Here's the drawing with two shaded views (mm, measured from the low corner). I have some questions. A direction names the side the tool comes from. Give positions to 0.01 mm unless a question says otherwise; leave off trailing zeros. Loops run counter-clockwise (first coordinate to the right, second up) from the corner with the lowest first, then second, coordinate; pieces in that order, holes last. Notation, with made-up numbers: M -2,33 L 55,33 A14 ccw 55,51 Z; hole C 72,-31 d9. An arc over 180 degrees is marked long. Use a Markdown table: item, result. Add a question column.
1) Will this pin go through, and if not, where does the flat tip stop? pin 1 Ø1.9 at (x, y) = (53.5, 2) entering from -Z.
2) If I drill on line 1 along X through (y, z) = (4.25, 4.75); line 2 along Z through (x, y) = (41, 1), over which ranges is the centre line in solid material (lowest first)? Write a range as [from, to].
3) Suppose I cut it at A-A on y = 5.25. List the corners of the cut face in (x, z) for me, and give its area (3 significant figures).
4) Which directions (+Z, -Z, +X, -X, +Y, -Y) give clear straight access to the entire face, cutting with the end or side of a thin tool? Please do the marked faces 1 and 2.
5) Suppose I cut it at B-B on x = 37. List the corners of the cut face in (y, z) for me, and give its area (3 significant figures).
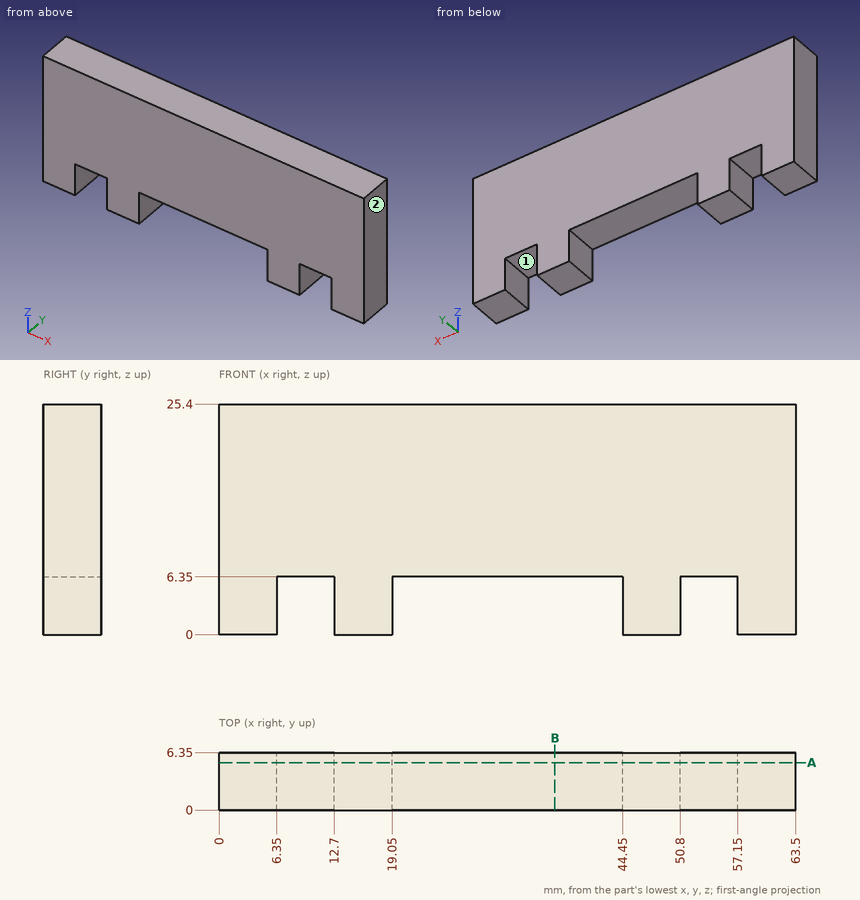
Answer block:
| question | item | result |
|---|---|---|
| 1 | pin 1 | stops at z = 6.35 |
| 2 | line 1 | x = [0, 6.35], [12.7, 19.05], [44.45, 50.8], [57.15, 63.5] |
| 2 | line 2 | z = [6.35, 25.4] |
| 3 | outline | M 0,0 L 6.35,0 L 6.35,6.35 L 12.7,6.35 L 12.7,0 L 19.05,0 L 19.05,6.35 L 44.45,6.35 L 44.45,0 L 50.8,0 L 50.8,6.35 L 57.15,6.35 L 57.15,0 L 63.5,0 L 63.5,25.4 L 0,25.4 Z |
| 3 | area | 1,370 mm^2 |
| 4 | face 1 | -Z, +Y, -Y |
| 4 | face 2 | +Z, -Z, +X, +Y, -Y |
| 5 | outline | M 0,6.35 L 6.35,6.35 L 6.35,25.4 L 0,25.4 Z |
| 5 | area | 121 mm^2 |
